For this review, take the finished solid that the model builds, in its own axes (mm). Face numbers are marked on the shaded views. A direction names the side the tool comes from. Give positions to 0.01 mm unless a question says otherwise; leave off trailing zeros. Order: outer loops, then holes, each group sorted by start corner. A loop starts at its lowest first (then second) coordinate and runs counter-clockwise, first axis right, second up. Notation, with made-up numbers: (80.25, -26) - (103.25, -26) arc R29 cw to (103.25, 5) - close; hole circle Ø11 at (-21.75, -17.5). An arc over 180 degrees is marked (long way). One line per item, written item: value.
```python
from build123d import *

# Parameters (mm, degrees)
SKETCH5_W           = 1000
SKETCH5_H           = 1000
BOSS_EXTRUDE1_DEPTH = 30
BOSS_EXTRUDE2_DEPTH = 940
SKETCH7_W           = 1250
SKETCH7_H           = 1500
BOSS_EXTRUDE3_DEPTH = 30
BOSS_EXTRUDE4_DEPTH = 445
CUT_EXTRUDE2_DEPTH  = 30
CUT_EXTRUDE3_DEPTH  = 30
SKETCH12_W          = 20
SKETCH12_H          = 850
BOSS_EXTRUDE5_DEPTH = 320
CUT_EXTRUDE4_DEPTH  = 700
BOSS_EXTRUDE6_DEPTH = 210
BOSS_EXTRUDE7_DEPTH = 490


with BuildPart() as part:
    # Sketch5 → Boss-Extrude1 (new body)
    with BuildSketch(Plane(origin=(0, 0, 0), x_dir=(1, 0, 0), z_dir=(0, 1, 0))):
        with Locations((-269.230769231, -730.850115694)):
            Rectangle(SKETCH5_W, SKETCH5_H)
    extrude(amount=BOSS_EXTRUDE1_DEPTH)

    # Sketch6 → Boss-Extrude2 (add)
    with BuildSketch(Plane.XZ):
        Polygon((-644.230769231, 625.850115694), (-644.230769231, 605.850115694), (-524.088400017, 605.850115694), (-524.088400017, 355.850115694), (-644.088400017, 355.850115694), (-644.088400017, 335.850115694), (-394.088400017, 335.850115694), (-394.088400017, 355.850115694), (-514.088400017, 355.850115694), (-514.088400017, 605.850115694), (-394.230769231, 605.850115694), (-394.230769231, 625.850115694), align=None)
        Polygon((-644.230769231, 1125.850115694), (-644.230769231, 1105.850115694), (-524.088400017, 1105.850115694), (-524.088400017, 855.850115694), (-644.088400017, 855.850115694), (-644.088400017, 835.850115694), (-394.088400017, 835.850115694), (-394.088400017, 855.850115694), (-514.088400017, 855.850115694), (-514.088400017, 1105.850115694), (-394.230769231, 1105.850115694), (-394.230769231, 1125.850115694), align=None)
        Polygon((-144.230769231, 1125.850115694), (-144.230769231, 1105.850115694), (-24.088400017, 1105.850115694), (-24.088400017, 855.850115694), (-144.088400017, 855.850115694), (-144.088400017, 835.850115694), (105.911599983, 835.850115694), (105.911599983, 855.850115694), (-14.088400017, 855.850115694), (-14.088400017, 1105.850115694), (105.769230769, 1105.850115694), (105.769230769, 1125.850115694), align=None)
        Polygon((-144.230769231, 625.850115694), (-144.230769231, 605.850115694), (-24.088400017, 605.850115694), (-24.088400017, 355.850115694), (-144.088400017, 355.850115694), (-144.088400017, 335.850115694), (105.911599983, 335.850115694), (105.911599983, 355.850115694), (-14.088400017, 355.850115694), (-14.088400017, 605.850115694), (105.769230769, 605.850115694), (105.769230769, 625.850115694), align=None)
    extrude(amount=BOSS_EXTRUDE2_DEPTH)

    # Sketch7 → Boss-Extrude3 (add)
    with BuildSketch(Plane.XZ.offset(940)):
        with Locations((-394.230769231, 730.850115694)):
            Rectangle(SKETCH7_W, SKETCH7_H)
    extrude(amount=BOSS_EXTRUDE3_DEPTH)

    # Sketch8 → Boss-Extrude4 (add)
    with BuildSketch(Plane.ZY.offset(524.088400017)):
        Polygon((480.850115694, -100), (470.850115694, -100), (470.850115694, -940), (490.850115694, -940), (490.850115694, -100), align=None)
        Polygon((975.850115694, -100), (970.850115694, -100), (970.850115694, -940), (990.850115694, -940), (990.850115694, -100), align=None)
    extrude(amount=BOSS_EXTRUDE4_DEPTH)

    # Sketch10 → Cut-Extrude2 (cut)
    with BuildSketch(Plane(origin=(0, 0, 470.850115694), x_dir=(-1, 0, 0), z_dir=(0, 0, -1))):
        Polygon((524.088400017, -100), (969.088400017, -940), (969.088400017, -100), align=None)
    extrude(amount=-CUT_EXTRUDE2_DEPTH, mode=Mode.SUBTRACT)

    # Sketch11 → Cut-Extrude3 (cut)
    with BuildSketch(Plane.XY.offset(990.850115694)):
        Polygon((-969.088400017, -100), (-524.088400017, -100), (-969.088400017, -940), align=None)
    extrude(amount=-CUT_EXTRUDE3_DEPTH, mode=Mode.SUBTRACT)

    # Sketch12 → Boss-Extrude5 (add)
    with BuildSketch(Plane.XY.offset(1125.850115694)):
        with Locations((-519.230769231, -515)):
            Rectangle(SKETCH12_W, SKETCH12_H)
        with Locations((-19.230769231, -515)):
            Rectangle(SKETCH12_W, SKETCH12_H)
    boss_extrude5 = extrude(amount=BOSS_EXTRUDE5_DEPTH)

    # Sketch13 → Cut-Extrude4 (cut)
    with BuildSketch(Plane.ZY.offset(529.230769231)):
        Polygon((1125.850115694, -90), (1445.850115694, -940), (1445.850115694, -90), align=None)
    cut_extrude4 = extrude(amount=-CUT_EXTRUDE4_DEPTH, mode=Mode.SUBTRACT)

    # Mirror1: Boss-Extrude5 across plane
    add(boss_extrude5.mirror(Plane(origin=(0, 0, 730.850115694), x_dir=(1, 0, 0), z_dir=(0, 0, -1))))

    # Mirror2: Cut-Extrude4 across plane
    add(cut_extrude4.mirror(Plane(origin=(0, 0, 730.850115694), x_dir=(1, 0, 0), z_dir=(0, 0, -1))), mode=Mode.SUBTRACT)

    # Sketch15 → Boss-Extrude6 (add)
    with BuildSketch(Plane(origin=(0, 0, 835.850115694), x_dir=(-1, 0, 0), z_dir=(0, 0, -1))):
        Polygon((549.088400017, -495), (579.088400017, -495), (579.088400017, -440), (459.088400017, -440), (459.088400017, -495), (489.088400017, -495), (489.088400017, -470), (549.088400017, -470), align=None)
    extrude(amount=BOSS_EXTRUDE6_DEPTH)

    # Sketch18 → Boss-Extrude7 (add)
    with BuildSketch(Plane(origin=(-514.088400017, 0, 0), x_dir=(0, 0, -1), z_dir=(1, 0, 0))):
        Polygon((-950.850115694, -495), (-920.850115694, -495), (-920.850115694, -440), (-1040.850115694, -440), (-1040.850115694, -495), (-1010.850115694, -495), (-1010.850115694, -470), (-950.850115694, -470), align=None)
    boss_extrude7 = extrude(amount=BOSS_EXTRUDE7_DEPTH)

    # Mirror3: Boss-Extrude7 across plane
    add(boss_extrude7.mirror(Plane(origin=(0, 0, 730.850115694), x_dir=(1, 0, 0), z_dir=(0, 0, -1))))


solid = part.part
```
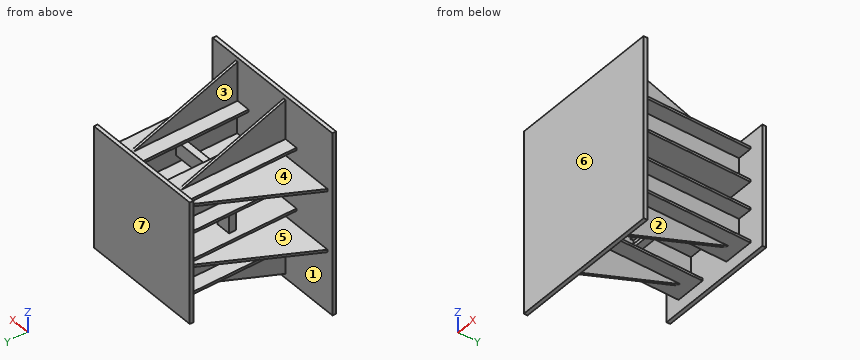
(1) Take a section at C-C (z = 282). Write out the cut boundary in (x, y).
Answers below:
outline: (-1019.23, -970) - (230.77, -970) - (230.77, -940) - (-9.23, -940) - (-9.23, -233.04) - (-29.23, -233.04) - (-29.23, -940) - (-509.23, -940) - (-509.23, -233.04) - (-529.23, -233.04) - (-529.23, -940) - (-1019.23, -940) - close; (-769.23, 0) - (230.77, 0) - (230.77, 30) - (-769.23, 30) - close
(2) Take a section at B-B (x = -272). Write out the cut boundary in (y, z).
Answers below:
outline: (-970, -19.15) - (-940, -19.15) - (-940, 1480.85) - (-970, 1480.85) - close; (-495, 420.85) - (-440, 420.85) - (-440, 540.85) - (-495, 540.85) - (-495, 510.85) - (-470, 510.85) - (-470, 450.85) - (-495, 450.85) - close; (-495, 920.85) - (-440, 920.85) - (-440, 1040.85) - (-495, 1040.85) - (-495, 1010.85) - (-470, 1010.85) - (-470, 950.85) - (-495, 950.85) - close; (0, 230.85) - (30, 230.85) - (30, 1230.85) - (0, 1230.85) - close
(3) Draft analysis for pull direction Y (two halves, no side actions). For the marked faces 5, 6 and 7, state which applies: pulls with the +Y half, pulls with the -Y half, needs draft (parallel to the pull), parting line crosses it, or undercut.
Answers below:
face 5: undercut
face 6: pulls with the -Y half
face 7: pulls with the +Y half
(4) Take a section at A-A (z = 809). Write out the cut boundary in (x, y).
Answers below:
outline: (-1019.23, -970) - (230.77, -970) - (230.77, -940) - (-1019.23, -940) - close; (-769.23, 0) - (230.77, 0) - (230.77, 30) - (-769.23, 30) - close; (-579.09, -495) - (-549.09, -495) - (-549.09, -470) - (-489.09, -470) - (-489.09, -495) - (-459.09, -495) - (-459.09, -440) - (-579.09, -440) - close
(5) For P1, Ø10, axis at y = -143, z = 1031, coming from the -X side; P2, Ø16.5, axis at x = -152, y = -472, coming from the +Z side; P3, Ø10, axis at x = -350, z = 159.5, coming from the +Y side, all flat-tipped, find the tip position at first contact; note any pin that passes through.
Answers below:
P1: stops at x = -524.09
P2: stops at z = 1125.85
P3: stops at y = -940
(6) Take a section at D-D (x = -610.5). Give the number of separate pieces and of enclosed holes in the cut face, then the cut area to 3 significant figures.
Answers below:
separate pieces: 1
enclosed holes: 3
area: 177,000 mm^2
(7) Machinability: for the marked faces 1, 2, 3 and 4, which of the approach directions +Z, -Z, +X, -X, +Y, -Y give a long, thin tool a straight path to every point of the face, cutting with its end or side? Answer none if there is none.
Answers below:
face 1: none
face 2: -Z, +X
face 3: +Z
face 4: -X
(8) Wall thickness on line 1 (Z direction, x = 81.5, y = -252); line 2 (Y direction, x = -75, z = 988); line 3 (Z direction, x = -622, y = -722): over which ranges is each line inside the solid? List them lowest first. Write a range as from..to.
Answers below:
line 1: z = 335.85..355.85, 605.85..625.85, 835.85..855.85, 1105.85..1125.85
line 2: y = -970..-940, -470..-440, 0..30
line 3: z = 335.85..355.85, 470.85..490.85, 605.85..625.85, 835.85..855.85, 970.85..990.85, 1105.85..1125.85
